Can you work these out from the model? Positions are in its coordinate system, mm. Give positions to 0.01 mm unless a question says otherwise; leave off trailing zeros. Order: outer loops, then holes, each group sorted by start corner. A loop starts at its lowest first (then second) coordinate and runs counter-clockwise, first axis right, second up. Notation, with made-up numbers: (26.5, -32.5) - (80.5, -32.5) arc R21 cw to (80.5, -3.5) - close; hole circle Ø9 at (14, -15). An arc over 180 degrees is marked (long way). Answer as CSV lines item,"result".
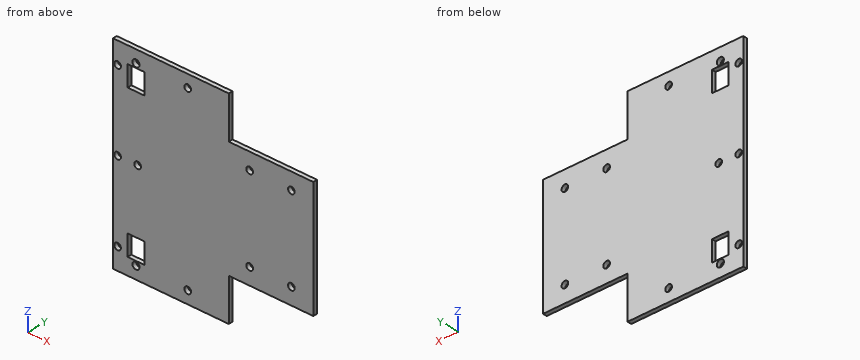
Autodesk Inventor part; units mm, degrees
ref_plane "YZ Plane" through (0, 0, 0) normal (1, 0, 0) x (0, 1, 0)
ref_plane "XZ Plane" through (0, 0, 0) normal (0, 1, 0) x (-1, 0, 0)
ref_plane "XY Plane" through (0, 0, 0) normal (0, 0, 1) x (1, 0, 0)
sketch "Szkic1" plane through (0, 0, 0) normal (0, 1, 0) x (-1, 0, 0)
  line L0 (40.5, 0) -> (96, 0)
  line L1 (96, 0) -> (96, -98)
  line L2 (96, -98) -> (40.5, -98)
  line L3 (0, -77.5) -> (0, -20.5)
  line L4 (40.5, 0) -> (40.5, -20.5)
  line L5 (40.5, -20.5) -> (0, -20.5)
  line L6 (40.5, -98) -> (40.5, -77.5)
  line L7 (40.5, -77.5) -> (0, -77.5)
  line L8 (0, -49) -> (96, -49) construction
  line L9 (10.5, -77.5) -> (10.5, -20.5) construction
  line L10 (30.5, -77.5) -> (30.5, -20.5) construction
  line L11 (93.8, 0) -> (93.8, -98) construction
  line L12 (96, -6) -> (40.5, -6) construction
  line L13 (96, -92) -> (40.5, -92) construction
  line L14 (84.2, 0) -> (84.2, -98) construction
  line L15 (85, 0) -> (85, -98) construction
  line L16 (89, -8) -> (81, -8)
  line L17 (81, -8) -> (81, -18)
  line L18 (81, -18) -> (89, -18)
  line L19 (89, -18) -> (89, -8)
  line L20 (89, -90) -> (81, -90)
  line L21 (81, -90) -> (81, -80)
  line L22 (81, -80) -> (89, -80)
  line L23 (89, -80) -> (89, -90)
  point P0 (0, 0)
  point P1 (30.5, -28.5)
  point P2 (30.5, -69.5)
  point P3 (10.5, -28.5)
  point P4 (10.5, -69.5)
  point P5 (93.8, -10.4)
  point P6 (93.8, -87.6)
  point P7 (93.8, -49)
  point P8 (60.2, -6)
  point P9 (60.2, -92)
  point P10 (84.2, -49)
  point P11 (85, -6)
  point P12 (85, -92)
  dimension "d0" = 98
  dimension "d2" = 20.5
  dimension "d3" = 40.5
  dimension "d12" = 96
  dimension "d42" = 57
  dimension "d71" = 10.4
  dimension "d72" = 6
  dimension "d73" = 2.2
  dimension "d81" = 35.8
  dimension "d89" = 30.5
  dimension "d90" = 8
  dimension "d91" = 8
  dimension "d92" = 8
  dimension "d93" = 11.8
  dimension "d94" = 11
  dimension "d95" = 10.5
  dimension "d96" = 6
  dimension "d97" = 0
  dimension "d98" = 96
  dimension "d106" = 8
  dimension "d107" = 10
  dimension "d108" = 7
  dimension "d109" = 8
extrude "Wyciągnięcie proste1" add sketch "Szkic1" along normal blind 2 contours L0 L1 L2 L6 L7 L3 L5 L4 | L19 L18 L17 L16 | L20 L21 L22 L23
hole "Hole4" at (-30.5, 0, -28.5) at (-30.5, 0, -69.5) at (-10.5, 0, -28.5) at (-10.5, 0, -69.5) direction (0, 1, 0) diameter 3.2 depth 10
hole "Otwór5" at (-93.8, 0, -10.4) at (-93.8, 0, -87.6) at (-93.8, 0, -49) direction (0, 1, 0) diameter 3.2 end through all
hole "Hole6" at (-60.2, 0, -6) at (-60.2, 0, -92) direction (0, 1, 0) diameter 3.2 depth 30
hole "Hole7" at (-84.2, 0, -49) direction (0, 1, 0) diameter 3.2 depth 30
hole "Hole8" at (-85, 0, -6) at (-85, 0, -92) direction (0, 1, 0) diameter 3.4 end through all
extrude "Extrusion2" cut sketch "Szkic1" along normal blind 10 contours L19 L18 L17 L16 | L20 L21 L22 L23
properties part number "PodstawaPEM"
1) I want a section at B-B on z = -49. Write out the boundary of the cut face in (x, y), plus the area to 3 significant figures.
Answer block:
outline,"(-96, 0) - (-95.4, 0) - (-95.4, 2) - (-96, 2) - close; (-92.2, 0) - (-85.8, 0) - (-85.8, 2) - (-92.2, 2) - close; (-82.6, 0) - (0, 0) - (0, 2) - (-82.6, 2) - close"
area,"179 mm2"
2) I want a section at C-C on y = 0.3. Count the separate pieces of the cut face and the enclosed holes in it, plus the area to 3 significant figures.
Answer block:
separate pieces,"1"
enclosed holes,"14"
area,"7,490 mm2"
3) I want a section at D-D on x = -93.8. Write out the boundary of the cut face in (y, z).
Answer block:
outline,"(0, -98) - (2, -98) - (2, -89.2) - (0, -89.2) - close; (0, -86) - (2, -86) - (2, -50.6) - (0, -50.6) - close; (0, -47.4) - (2, -47.4) - (2, -12) - (0, -12) - close; (0, -8.8) - (2, -8.8) - (2, 0) - (0, 0) - close"
4) I want a section at A-A on x = -60.2. Write out the boundary of the cut face in (y, z), plus the area to 3 significant figures.
Answer block:
outline,"(0, -98) - (2, -98) - (2, -93.6) - (0, -93.6) - close; (0, -90.4) - (2, -90.4) - (2, -7.6) - (0, -7.6) - close; (0, -4.4) - (2, -4.4) - (2, 0) - (0, 0) - close"
area,"183 mm2"
5) I need wall thicknesses on line 1 along X through (y, z) = (1.55, -69.5); line 2 along Z through (x, y) = (-93.8, 0.65); line 3 along X through (y, z) = (0.4, -49). Which ranges of each line are inside material? Lowest first, please. Write a range as [from, to].
Answer block:
line 1,"[-96, -32.1], [-28.9, -12.1], [-8.9, 0]"
line 2,"[-98, -89.2], [-86, -50.6], [-47.4, -12], [-8.8, 0]"
line 3,"[-96, -95.4], [-92.2, -85.8], [-82.6, 0]"
6) I'm going to push flat-ended pins straight in: P1, Ø1, axis at x = -36, y = 1, coming from the +Z side; P2, Ø0.6, axis at y = 1, z = -15, coming from the +X side. Where does each tip first touch, or does it pass through?
Answer block:
P1,"z = -20.5"
P2,"x = -40.5"
